Input: part model. Units: mm. Frame: model coordinates. A direction names the side the tool comes from. Coordinates: 2 decimals unless noted, no trailing zeros. Order: outer loops, then holes, each group sorted by start corner. A loop starts at its lowest first (then second) coordinate and runs counter-clockwise, first axis right, second up. Notation, with made-up numbers: (66.5, -35) - (111.5, -35) arc R10 cw to (111.5, -27) - close; hole circle Ø6 at (-36, 74.5). An arc over 180 degrees is marked (long way). One line per question, with ' | ' between items.
from build123d import *

# Parameters (mm, degrees)
SKETCH_1_W                     = 88.5
SKETCH_1_H                     = 25
EXTRUDE_1_DEPTH                = 8
CUT_EXTRUDE_2_DEPTH            = 70
SKETCH_9_W                     = 16.75
SKETCH_9_H                     = 7.5
CUT_EXTRUDE_3_DEPTH            = 6
FILLET_4_R                     = 2
PATTERN_LINEAR_1_COUNT         = 4
PATTERN_LINEAR_1_PITCH         = 18.5
PATTERN_LINEAR_1_COUNT_DIR2    = 2
PATTERN_LINEAR_1_PITCH_DIR2    = 9.5
FILLET_4_OF_PATTERN_LINEAR_1_R = 2
SKETCH_10_W                    = 8
SKETCH_10_H                    = 25
EXTRUDE_2_DEPTH                = 110
FILLET_5_R                     = 20
FILLET_6_R                     = 15
FILLET_7_R                     = 5
CUT_EXTRUDE_4_DEPTH            = 95
CUT_EXTRUDE_5_REACH            = 145.378
CUT_EXTRUDE_7_REACH            = 145.378


with BuildPart() as part:
    # Эскиз1 → Бобышка-Вытянуть1 (new body)
    with BuildSketch(Plane.XY):
        with Locations((44.25, 12.5)):
            Rectangle(SKETCH_1_W, SKETCH_1_H)
    extrude(amount=EXTRUDE_1_DEPTH)

    # Эскиз4 → Вырез-Вытянуть2 (cut)
    with BuildSketch(Plane.ZY):
        Polygon((6, 0), (0, 3.464101615), (0, 0), align=None)
        Polygon((0, 25), (6, 25), (0, 21.535898385), align=None)
    extrude(amount=-CUT_EXTRUDE_2_DEPTH, mode=Mode.SUBTRACT)

    # Эскиз9 → Вырез-Вытянуть3 (cut)
    with BuildSketch(Plane.XY.offset(8)):
        with Locations((13.928226592, 17.25)):
            Rectangle(SKETCH_9_W, SKETCH_9_H)
    cut_extrude_3 = extrude(amount=-CUT_EXTRUDE_3_DEPTH, mode=Mode.SUBTRACT)

    # Скругление4
    fillet_4_edges = [part.edges().sort_by_distance(p)[0] for p in [
        (22.303226592, 13.5, 5),
        (22.303226592, 21, 5),
        (5.553226592, 21, 5),
        (5.553226592, 13.5, 5),
    ]]
    fillet(fillet_4_edges, radius=FILLET_4_R)

    # Линейный массив1: Cut-Extrude 3 4 × 2
    with Locations(*[(i * PATTERN_LINEAR_1_PITCH, -j * PATTERN_LINEAR_1_PITCH_DIR2, 0) for i in range(PATTERN_LINEAR_1_COUNT) for j in range(PATTERN_LINEAR_1_COUNT_DIR2) if (i, j) != (0, 0)]):
        add(cut_extrude_3, mode=Mode.SUBTRACT)

    # Скругление4 of Линейный массив1
    fillet_4_of_pattern_linear_1_edges = [part.edges().sort_by_distance(p)[0] for p in [
        (22.303226592, 4, 5),
        (22.303226592, 11.5, 5),
        (5.553226592, 11.5, 5),
        (5.553226592, 4, 5),
        (40.803226592, 13.5, 5),
        (40.803226592, 21, 5),
        (24.053226592, 21, 5),
        (24.053226592, 13.5, 5),
        (40.803226592, 4, 5),
        (40.803226592, 11.5, 5),
        (24.053226592, 11.5, 5),
        (24.053226592, 4, 5),
        (59.303226592, 13.5, 5),
        (59.303226592, 21, 5),
        (42.553226592, 21, 5),
        (42.553226592, 13.5, 5),
        (59.303226592, 4, 5),
        (59.303226592, 11.5, 5),
        (42.553226592, 11.5, 5),
        (42.553226592, 4, 5),
        (77.803226592, 13.5, 5),
        (77.803226592, 21, 5),
        (61.053226592, 21, 5),
        (61.053226592, 13.5, 5),
        (77.803226592, 4, 5),
        (77.803226592, 11.5, 5),
        (61.053226592, 11.5, 5),
        (61.053226592, 4, 5),
    ]]
    fillet(fillet_4_of_pattern_linear_1_edges, radius=FILLET_4_OF_PATTERN_LINEAR_1_R)

    # Эскиз10 → Бобышка-Вытянуть2 (add)
    with BuildSketch(Plane(origin=(0, 0, 0), x_dir=(-1, 0, 0), z_dir=(0, 0, -1))):
        with Locations((-84.5, 12.5)):
            Rectangle(SKETCH_10_W, SKETCH_10_H)
    extrude(amount=EXTRUDE_2_DEPTH)

    # Скругление5
    # the kernel refuses this fillet: 20 mm, written as the material it takes off along each edge
    with BuildSketch(Plane(origin=(88.5, -50, 8), x_dir=(-1, 0, 0), z_dir=(0, 1, 0))) as fillet_5_piece_1:
        with BuildLine():
            CenterArc((FILLET_5_R, -FILLET_5_R), FILLET_5_R, 90, 90)
            Line((0, -FILLET_5_R), (0, 0))
            Line((0, 0), (FILLET_5_R, 0))
        make_face()
    extrude(amount=125, mode=Mode.SUBTRACT)

    # Скругление6
    fillet_6_edges = [part.edges().sort_by_distance(p)[0] for p in [
        (80.5, 12.5, 0),
    ]]
    fillet(fillet_6_edges, radius=FILLET_6_R)

    # Скругление7
    fillet_7_edges = [part.edges().sort_by_distance(p)[0] for p in [
        (84.5, 0, -110),
        (84.5, 25, -110),
    ]]
    fillet(fillet_7_edges, radius=FILLET_7_R)

    # Эскиз11 → Вырез-Вытянуть4 (cut)
    with BuildSketch(Plane(origin=(0, 0, -110), x_dir=(-1, 0, 0), z_dir=(0, 0, -1))):
        Polygon((-82.5, 25), (-88.5, 25), (-88.5, 21.535898385), align=None)
        Polygon((-88.5, 3.464101615), (-82.5, 0), (-88.5, 0), align=None)
    extrude(amount=-CUT_EXTRUDE_4_DEPTH, mode=Mode.SUBTRACT)

    # Эскиз12 → Вырез-Вытянуть5 (cut, up to next)
    with BuildSketch(Plane(origin=(88.5, 0, 0), x_dir=(0, 0, -1), z_dir=(1, 0, 0)), mode=Mode.PRIVATE) as cut_extrude_5_sk1:
        with BuildLine():
            Line((20, 17.5), (100, 17.5))
            ThreePointArc((100, 17.5), (105, 12.5), (100, 7.5))
            Line((100, 7.5), (20, 7.5))
            ThreePointArc((20, 7.5), (15, 12.5), (20, 17.5))
        make_face()
    cut_extrude_5_tool1 = extrude(cut_extrude_5_sk1.sketch, amount=-CUT_EXTRUDE_5_REACH, mode=Mode.PRIVATE) & part.part
    add(cut_extrude_5_tool1.solids().sort_by_distance((88.5, 12.5, -60))[0], mode=Mode.SUBTRACT)

    # Эскиз13 → Вырез-Вытянуть7 (cut, up to next)
    with BuildSketch(Plane(origin=(0, 0, 0), x_dir=(-1, 0, 0), z_dir=(0, 0, -1)), mode=Mode.PRIVATE) as cut_extrude_7_sk1:
        with BuildLine():
            Line((-3.30197377, 25), (0, 25))
            Line((0, 25), (0, 0))
            Line((0, 0), (-3.30197377, 0))
            ThreePointArc((-3.30197377, 0), (-0.1, 12.5), (-3.30197377, 25))
        make_face()
    cut_extrude_7_tool1 = extrude(cut_extrude_7_sk1.sketch, amount=-CUT_EXTRUDE_7_REACH, mode=Mode.PRIVATE) & part.part
    add(cut_extrude_7_tool1.solids().sort_by_distance((1.650987, 24.747829, 0))[0], mode=Mode.SUBTRACT)


solid = part.part
Item 1: Draft query along Y for faces 4 (the face through (59.303, 17, 5)), 5 (the face through (34, 13, 8)), 6 (the face through (84, 23, -109)). Return one class per face: released by +Y, released by -Y, zero draft, split by the parting line, or undercut.
Data:
face 4: undercut | face 5: zero draft | face 6: released by +Y
Item 2: Ray query, line 1 (Z direction, x = 19, y = 18); line 2 (X direction, y = 20, z = -32.5); line 3 (Z direction, x = 47.5, y = 13.25). Return the intervals inside material, ascending.
Data:
line 1: 0 to 2 | line 2: 80.5 to 88.5 | line 3: 0 to 8
Item 3: Contact query for flat-ended pins moving along their axis: P1, Ø1, axis at x = 85, y = 1.5, coming from the -Z side; P2, Ø4, axis at y = 18, z = 5, coming from the +X side; P3, Ø3, axis at x = 31.5, z = 4, coming from the +Y side. Output: stop coordinate, or through.
Data:
P1: z = -109 | P2: x = 81.73 | P3: y = 24.71
Item 4: Section C-C on y = 2.25. Return the cut outline in (x, z).
Data:
outline: (2.21, 2.1) - (70, 2.1) - (70, -0.69) arc R15 cw to (80.5, -15) - (80.5, -109.18) - (86.4, -109.18) - (86.4, -15) - (88.5, -15) - (88.5, -12) arc R20 ccw to (68.5, 8) - (2.21, 8) - close
Item 5: Section B-B on x = 28. Return the cut outline in (y, z), and give its area (3 significant figures).
Data:
outline: (0, 6) - (3.46, 0) - (21.54, 0) - (25, 6) - (25, 8) - (21, 8) - (21, 2) - (13.5, 2) - (13.5, 8) - (11.5, 8) - (11.5, 2) - (4, 2) - (4, 8) - (0, 8) - close | area: 89.2 mm^2
Item 6: Access query for faces 1 (the face through (84.6, 12.6, -105)), 2 (the face through (70, 1, 1)), 3 (the face through (69, 11.5, 5)). Directions: +Z, -Z, +X, -X, +Y, -Y. A direction counts if a zero-diameter tool reaches every point of the face in a straight line with its end or side. Return the directions, or none.
Data:
face 1: +X, -X | face 2: -Z, -X, -Y | face 3: +Z
Item 7: Section A-A on z = -45.5. Return the cut outline in (x, y).
Data:
outline: (80.5, 0) - (82.5, 0) - (88.5, 3.46) - (88.5, 7.5) - (80.5, 7.5) - close; (80.5, 17.5) - (88.5, 17.5) - (88.5, 21.54) - (82.5, 25) - (80.5, 25) - close
